Verification items for the finished model (mm, model axes). Face numbers are marked on the shaded views. A direction names the side the tool comes from. Give positions to 0.01 mm unless a question says otherwise; leave off trailing zeros. Write each loop counter-clockwise with the first axis right and the second up, starting at its lowest first coordinate (ties: lowest second). Pieces come first, ordered by that corner, then holes. Notation, with made-up numbers: (37.5, 85.25) - (54.5, 85.25) arc R25 cw to (54.5, 122.25) - close; hole circle Ø11 at (64.25, 34.25). An arc over 180 degrees is marked (long way). Answer as a JSON object with one key per item and string values. Group by question number.
Item 1: Scan lines: line 1 along X through (y, z) = (-15.5, -3.3); line 2 along Z through (x, y) = (-19, 18.5). Record each from-to range of solid material in increasing order. Write a range as [from, to].
Item 2: Draft check along Z on the marked faces 1, 2 and 3. Enter one of: +Z half, -Z half, draft (parallel to the pull), parting line (faces both ways), or undercut.
Item 3: Tool access check on the marked faces 4, 5 and 6. Record the directions out of +Z, -Z, +X, -X, +Y, -Y that give a thin tool (end or side, any length) a straight path to the whole face; none if there is none.
Item 4: Sectioned sample at A-A, the plane z = -4. Record the boundary of the cut face in (x, y), and give its area (3 significant figures).
Item 5: Sectioned sample at B-B, the plane x = 0. Record the boundary of the cut face in (y, z), and give its area (3 significant figures).
Item 6: Sectioned sample at D-D, the plane z = -27.5. Record the boundary of the cut face in (x, y), and give its area (3 significant figures).
Item 7: Go/stop test with flat-tipped pins: pin 1 (8 mm diameter, centred on x = 15, z = 0, fed in from +Y); pin 2 (4.5 mm diameter, centred on x = 7, z = -41.5, fed in from -Y); pin 3 (12 mm diameter, centred on x = -6.5, z = 10.5, fed in from +Y); pin 4 (10.5 mm diameter, centred on x = -2, y = -2, fed in from +Z). Record where each tip stops, or that it passes through.
```python
from build123d import *

# Parameters (mm, degrees)
F3_DEPTH       = 8
F6_DEPTH       = 29.9
F8_DEPTH       = 8.9
F9_R           = 11
F9_R_2         = 4.7
F10_DEPTH      = 2
F11_R          = 2.5
F12_DEPTH      = 22.4
F12_DEPTH_BACK = 10
F11_R_2        = 4.7
F13_DEPTH      = 3
F15_D          = 3
F15_DEPTH      = 5
F15_TIP        = 0.9012909285


with BuildPart() as f3:
    # F1 (on Top) → F3 (new body, through all)
    with BuildSketch(Plane.XY):
        with BuildLine():
            ThreePointArc((21, 16.4890873004), (18.8797510577, 18.8797510577), (16.4890873004, 21))
            Line((16.4890873004, 21), (-16.4890873004, 21))
            ThreePointArc((-16.4890873004, 21), (-18.8797510577, 18.8797510577), (-21, 16.4890873004))
            Line((-21, 16.4890873004), (-21, -16.4890873004))
            ThreePointArc((-21, -16.4890873004), (-18.8797510577, -18.8797510577), (-16.4890873004, -21))
            Line((-16.4890873004, -21), (16.4890873004, -21))
            ThreePointArc((16.4890873004, -21), (18.8797510577, -18.8797510577), (21, -16.4890873004))
            Line((21, -16.4890873004), (21, 16.4890873004))
        make_face()
    extrude(amount=-F3_DEPTH)

    # F5 (on offset) → F6 (join, through all)
    with BuildSketch(Plane.XY.offset(-37.9)):
        with BuildLine():
            ThreePointArc((-21.1, -13.6862156932), (-17.7837355468, -17.7837355468), (-13.6862156932, -21.1))
            Line((-13.6862156932, -21.1), (13.6862156932, -21.1))
            ThreePointArc((13.6862156932, -21.1), (17.7837355468, -17.7837355468), (21.1, -13.6862156932))
            Line((21.1, -13.6862156932), (21.1, 13.6862156932))
            ThreePointArc((21.1, 13.6862156932), (17.7837355468, 17.7837355468), (13.6862156932, 21.1))
            Line((13.6862156932, 21.1), (-13.6862156932, 21.1))
            ThreePointArc((-13.6862156932, 21.1), (-17.7837355468, 17.7837355468), (-21.1, 13.6862156932))
            Line((-21.1, 13.6862156932), (-21.1, -13.6862156932))
        make_face()
    extrude(amount=F6_DEPTH)

    # F7 (on offset) → F8 (join)
    with BuildSketch(Plane.XY.offset(-37.9)):
        with BuildLine():
            ThreePointArc((21, 16.4890873004), (18.8797510577, 18.8797510577), (16.4890873004, 21))
            Line((16.4890873004, 21), (-16.4890873004, 21))
            ThreePointArc((-16.4890873004, 21), (-18.8797510577, 18.8797510577), (-21, 16.4890873004))
            Line((-21, 16.4890873004), (-21, -16.4890873004))
            ThreePointArc((-21, -16.4890873004), (-18.8797510577, -18.8797510577), (-16.4890873004, -21))
            Line((-16.4890873004, -21), (16.4890873004, -21))
            ThreePointArc((16.4890873004, -21), (18.8797510577, -18.8797510577), (21, -16.4890873004))
            Line((21, -16.4890873004), (21, 16.4890873004))
        make_face()
    extrude(amount=-F8_DEPTH)

    # F9 (on Top) → F10 (join)
    with BuildSketch(Plane.XY):
        Circle(F9_R)
        Circle(F9_R_2, mode=Mode.SUBTRACT)
    extrude(amount=F10_DEPTH)

    # F11 (on face) → F12 (join, two sides)
    with BuildSketch(Plane.XY.offset(2)) as f12_sk:
        Circle(F11_R)
    extrude(amount=F12_DEPTH)
    extrude(f12_sk.sketch, amount=-F12_DEPTH_BACK)

    # F11 (on face) → F13 (cut)
    with BuildSketch(Plane.XY.offset(2)):
        Circle(F11_R_2)
        Circle(F11_R, mode=Mode.SUBTRACT)
    extrude(amount=-F13_DEPTH, mode=Mode.SUBTRACT)

    # F15
    with Locations(Plane.XY):
        with Locations((-15.5, 15.5), (15.5, 15.5), (15.5, -15.5), (-15.5, -15.5)):
            Hole(F15_D / 2, depth=F15_DEPTH)
            with Locations((0, 0, -(F15_DEPTH + F15_TIP / 2))):  # 118° drill point
                Cone(0, F15_D / 2, F15_TIP, mode=Mode.SUBTRACT)


solid = f3.part
```
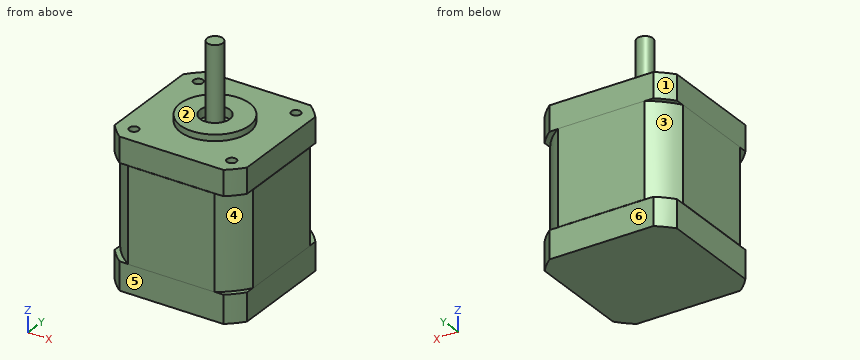
Geometry check:
{
 "1": {"line 1": "[-21, -17], [-14, 14], [17, 21]", "line 2": "[-46.8, -37.9], [-8, 0]"},
 "2": {"face 1": "draft", "face 2": "+Z half", "face 3": "undercut"},
 "3": {"face 4": "+X, -Y", "face 5": "-Z, +X, -X, -Y", "face 6": "-Z, +X, -X, +Y"},
 "4": {"outline": "(-21, -16.49) arc R26.7 ccw to (-16.49, -21) - (16.49, -21) arc R26.7 ccw to (21, -16.49) - (21, 16.49) arc R26.7 ccw to (16.49, 21) - (-16.49, 21) arc R26.7 ccw to (-21, 16.49) - close; hole circle Ø3 at (-15.5, -15.5); hole circle Ø3 at (-15.5, 15.5); hole circle Ø3 at (15.5, -15.5); hole circle Ø3 at (15.5, 15.5)", "area": "1,700 mm^2"},
 "5": {"outline": "(-21.1, -37.9) - (-21, -37.9) - (-21, -46.8) - (21, -46.8) - (21, -37.9) - (21.1, -37.9) - (21.1, -8) - (21, -8) - (21, 0) - (11, 0) - (11, 2) - (4.7, 2) - (4.7, -1) - (2.5, -1) - (2.5, 24.4) - (-2.5, 24.4) - (-2.5, -1) - (-4.7, -1) - (-4.7, 2) - (-11, 2) - (-11, 0) - (-21, 0) - (-21, -8) - (-21.1, -8) - close", "area": "2,110 mm^2"},
 "6": {"outline": "(-21.1, -13.69) arc R25.15 ccw to (-13.69, -21.1) - (13.69, -21.1) arc R25.15 ccw to (21.1, -13.69) - (21.1, 13.69) arc R25.15 ccw to (13.69, 21.1) - (-13.69, 21.1) arc R25.15 ccw to (-21.1, 13.69) - close", "area": "1,690 mm^2"},
 "7": {"pin 1": "y = 21", "pin 2": "y = -21", "pin 3": "y = 2.45", "pin 4": "z = 24.4"}
}
